from build123d import *

# Parameters (mm, degrees)
SKETCH_1_W          = 5
SKETCH_1_H          = 60
EXTRUDE_1_DEPTH     = 60
SKETCH_2_R          = 5
SKETCH_3_R          = 3.5
CUT_EXTRUDE_4_DEPTH = 137.839321834


with BuildPart() as part:
    # Эскиз1 → Вытянуть-Тонкостенный1 (new, symmetric)
    with BuildSketch(Plane.XY):
        with Locations((2.5, 30)):
            Rectangle(SKETCH_1_W, SKETCH_1_H)
    extrude(amount=EXTRUDE_1_DEPTH, both=True)

    # По траектории1: sweep along a curve in space
    with BuildLine() as sweep_1_path:
        Line((5, 60, 60), (5, 60, -60))
    # Эскиз2 → По траектории1 (sweep)
    with BuildSketch(Plane.XY.offset(60)):
        with Locations((5, 60)):
            Circle(SKETCH_2_R)
    sweep(path=sweep_1_path.line)

    # Эскиз3 → Вырез-Вытянуть4 (cut, through all)
    with BuildSketch(Plane.XY.offset(60)):
        with Locations((5, 60)):
            Circle(SKETCH_3_R)
    extrude(amount=-CUT_EXTRUDE_4_DEPTH, mode=Mode.SUBTRACT)


solid = part.part
For this review, take the finished solid that the model builds, in its own axes (mm). Round coordinates to 2 decimals unless told otherwise and drop trailing zeros. Write each loop counter-clockwise with the first axis right and the second up, starting at its lowest first coordinate (ties: lowest second). Pieces come first, ordered by that corner, then holes. Notation, with made-up numbers: (-7.5, -19) - (39.5, -19) arc R20 ccw to (39.5, -15) - close; hole circle Ø7 at (75, -31.75). An arc over 180 degrees is marked (long way). Write item = value, one per line. Start each with the question number.
1. Consider section C-C on y = 31. State the section outline as (x, z) points, plus the area to 3 significant figures.
2. Consider section B-B on x = 2.75. State the section outline as (y, z) points.
3. Wall thickness on L1, parallel to Y at x = 4.75, z = -26; L2, parallel to X at y = 20, z = 2; L3, parallel to Y at x = 4, z = 40: over which ranges is each line inside the solid? List them lowest first.
4. For pin 1 Ø2 at (y, z) = (30, 38.5) entering from +X, flat-tipped, find the tip position at first contact; note if it passes through.
5. Draft analysis for pull direction X (two halves, no side actions). For faces 1 (the face through (5, 27, 1)), 2 (the face through (0, 30, 1)), 3 (the face through (8.34, 61.05, 0.84)), 4 (the face through (8, 64, -1)), state which applies: released by +X, released by -X, zero draft, split by the parting line, or undercut.
6. Consider section A-A on z = -8. State the section outline as (x, y) points, plus the area to 3 significant figures.
Evaluation:
q1.outline = (0, -60) - (5, -60) - (5, 60) - (0, 60) - close
q1.area = 600 mm2
q2.outline = (0, -60) - (57.32, -60) - (57.32, 60) - (0, 60) - close; (62.68, -60) - (64.47, -60) - (64.47, 60) - (62.68, 60) - close
q3.L1 = 0 to 56.51, 63.49 to 64.99
q3.L2 = 0 to 5
q3.L3 = 0 to 56.65, 63.35 to 64.9
q4.pin_1 = 5
q5.face_1 = released by +X
q5.face_2 = released by -X
q5.face_3 = undercut
q5.face_4 = split by the parting line
q6.outline = (0, 0) - (5, 0) - (5, 55) arc R5 ccw (long way) to (0, 60) - close; hole circle Ø7 at (5, 60)
q6.area = 320 mm2
